Part model, mm, in its own coordinate system. Face numbers are marked on the shaded views. A direction names the side the tool comes from. Give positions to 0.01 mm unless a question says otherwise; leave off trailing zeros. Order: outer loops, then holes, each group sorted by start corner. A loop starts at its lowest first (then second) coordinate and runs counter-clockwise, first axis right, second up. Notation, with made-up numbers: (38, 68) - (47, 68) arc R23 cw to (47, 85) - close; hole circle Ø9 at (43, -29). An arc over 180 degrees is marked (long way). Use one line per item in the form item = value. Start each with the question number.
1. Band-saw the part on C-C, the plane y = -213. List the corners of the cut face in (x, z), plus the area to 3 significant figures.
2. Pin check, flat tips, straight feed: P1, Ø5.5, axis at x = 197.55, z = 3.2, coming from the -Y side; P2, Ø14.5, axis at x = 167.5, y = -180.5, coming from the +Z side; P3, Ø3, axis at y = -223.5, z = 9, coming from the -X side; P4, Ø8.5, axis at x = 88.5, z = 4.5, coming from the -Y side. Stop position of each tip, or through.
3. Band-saw the part on A-A, the plane x = 31. List the corners of the cut face in (y, z), plus the area to 3 significant figures.
4. Band-saw the part on B-B, the plane z = 8.5. State how many separate pieces and enclosed holes the cut face has, plus the area to 3 significant figures.
5. Pull direction X, two halves, no side cores. Call the marked faces 1, 2, 3 and 4: +X half, -X half, draft (parallel to the pull), parting line (faces both ways), or undercut.
6. Drill centre lines: line 1 (Z direction, x = 31, y = -188); line 2 (Z direction, x = 148.35, y = -226.6); line 3 (Y direction, x = 75, z = 7.5). Where is each one in solid material? Low to high.
7. Band-saw the part on D-D, the plane z = 20.25. List the corners of the cut face in (x, y), plus the area to 4 significant figures.
8. Tool access for the marked faces 5 and 6: list every direction of +Z, -Z, +X, -X, +Y, -Y with a clear straight run to the whole face (end or side of a thin tool).
from build123d import *

# Parameters (mm, degrees)
PAD067_DEPTH           = 10
PAD068_DEPTH           = 6
PAD072_DEPTH           = 14
CYLINDER038_R          = 2.2
CYLINDER038_DEPTH      = 26
CYLINDER038_ROLL_ANGLE = -90
ARRAY012_X_COUNT       = 2
ARRAY012_X_PITCH       = 8
ARRAY012_Z_COUNT       = 2
ARRAY012_Z_PITCH       = 9
BOX047_W               = 24
BOX047_H               = 10
BOX047_DEPTH           = 17
SKETCH056_R            = 3
PAD057_DEPTH           = 9
BOX048_W               = 35
BOX048_H               = 15
BOX048_DEPTH           = 20
BOX044_W               = 23
BOX044_H               = 3
BOX044_DEPTH           = 20
SKETCH049_R            = 3
PAD050_DEPTH           = 4
SKETCH050_R            = 3
PAD051_DEPTH           = 4
BOX043_W               = 20
BOX043_H               = 17
BOX043_DEPTH           = 10
FILLET017_R            = 1
FILLET017_ROLL_ANGLE   = 90
FILLET018_1_R          = 2
FILLET018_2_R          = 1
BOX042_W               = 167
BOX042_H               = 10
BOX042_DEPTH           = 17
CYLINDER037_R          = 2.2
CYLINDER037_DEPTH      = 18
CYLINDER037_ROLL_ANGLE = -90
ARRAY011_X_COUNT       = 2
ARRAY011_X_PITCH       = 49.2
ARRAY011_Z_COUNT       = 2
ARRAY011_Z_PITCH       = 10.3
PAD053_DEPTH           = 6
PAD052_DEPTH           = 10
CHAMFER007_SIZE        = 3
FILLET023_R            = 1
CHAMFER009_SIZE        = 7.5
PAD066_DEPTH           = 10


with BuildPart() as obj1:
    # Sketch067 → Pad067 (new body)
    with BuildSketch(Plane(origin=(142.7, 11, 18.5), x_dir=(0, 0, -1), z_dir=(1, 0, 0))):
        Polygon((0, 0), (0, 3), (3, 0), align=None)
    extrude(amount=PAD067_DEPTH)


with BuildPart() as obj2:
    # Sketch068 → Pad068 (new body)
    with BuildSketch(Plane(origin=(152.7, 45.8, 18.5), x_dir=(0, -1, 0), z_dir=(0, 0, 1))):
        Polygon((0, 0), (0, 3), (3, 0), align=None)
    extrude(amount=PAD068_DEPTH)


with BuildPart() as obj3:
    # Sketch065 → Pad072 (new body)
    with BuildSketch(Plane(origin=(152.7, 11, 17), x_dir=(1, 0, 0), z_dir=(0, -1, 0))):
        Polygon((0, 0), (0, 7), (7, 0), align=None)
    extrude(amount=PAD072_DEPTH)


with BuildPart() as obj4:
    # Cylinder038 → Cylinder038 (new body)
    with BuildSketch(Plane.XY):
        Circle(CYLINDER038_R)
    extrude(amount=CYLINDER038_DEPTH)


with BuildPart() as obj4_1:
    # Cylinder038 roll: moved
    add(obj4.part.rotate(Axis((0, 0, 0), (1, 0, 0)), CYLINDER038_ROLL_ANGLE))


with BuildPart() as obj4_2:
    # Cylinder038 placement: moved
    add(obj4_1.part.moved(Location((202, 0, 4))))

    # Array012 X: obj4_2


with BuildPart() as obj4_3:
    add(obj4_2.part)
    with Locations(*[(i * ARRAY012_X_PITCH, 0, 0) for i in range(1, ARRAY012_X_COUNT)]):
        add(obj4_2.part)

    # Array012 Z: obj4_2


with BuildPart() as obj4_4:
    add(obj4_3.part)
    with Locations(*[(0, 0, i * ARRAY012_Z_PITCH) for i in range(1, ARRAY012_Z_COUNT)]):
        add(obj4_3.part)


with BuildPart() as obj4_5:
    # Array012 placement: moved
    add(obj4_4.part.moved(Location((-171, -5, 0))))


with BuildPart() as obj5:
    # Box047 → Box047 (new body)
    with BuildSketch(Plane(origin=(26, 6, 0), x_dir=(1, 0, 0), z_dir=(0, 0, 1))):
        with Locations((12, 5)):
            Rectangle(BOX047_W, BOX047_H)
    extrude(amount=BOX047_DEPTH)


with BuildPart() as obj6:
    # Sketch056 → Pad057 (new body)
    with BuildSketch(Plane(origin=(50, 6, 0), x_dir=(1, 0, 0), z_dir=(0, -1, 0))):
        with BuildLine():
            Line((0, 17), (-36, 17))
            ThreePointArc((-36, 17), (-44.500015, 8.5), (-36, 0))
            Line((-36, 0), (0, 0))
            Line((0, 0), (0, 17))
        make_face()
        with Locations((-36.000015, 8.5)):
            Circle(SKETCH056_R, mode=Mode.SUBTRACT)
    extrude(amount=PAD057_DEPTH)


with BuildPart() as obj7:
    # Box048 → Box048 (new body)
    with BuildSketch(Plane(origin=(-2, -5, 0), x_dir=(1, 0, 0), z_dir=(0, 0, 1))):
        with Locations((17.5, 7.5)):
            Rectangle(BOX048_W, BOX048_H)
    extrude(amount=BOX048_DEPTH)


with BuildPart() as obj8:
    # Box044 → Box044 (new body)
    with BuildSketch(Plane(origin=(80.5, 1, 0), x_dir=(1, 0, 0), z_dir=(0, 0, 1))):
        with Locations((11.5, 1.5)):
            Rectangle(BOX044_W, BOX044_H)
    extrude(amount=BOX044_DEPTH)


with BuildPart() as obj9:
    # Sketch049 → Pad050 (new body)
    with BuildSketch(Plane.XY):
        with BuildLine():
            Line((0, 17), (20, 17))
            ThreePointArc((20, 0), (28.500019, 8.5), (20, 17))
            Line((20, 0), (0, 0))
            Line((0, 0), (0, 17))
        make_face()
        with Locations((20.000019, 8.5)):
            Circle(SKETCH049_R, mode=Mode.SUBTRACT)
    extrude(amount=PAD050_DEPTH)


with BuildPart() as obj10:
    # Sketch050 → Pad051 (new body)
    with BuildSketch(Plane.XY.offset(14)):
        with BuildLine():
            Line((0, 17), (20, 17))
            ThreePointArc((20, 0), (28.500019, 8.5), (20, 17))
            Line((20, 0), (0, 0))
            Line((0, 0), (0, 17))
        make_face()
        with Locations((20.000019, 8.5)):
            Circle(SKETCH050_R, mode=Mode.SUBTRACT)
    extrude(amount=PAD051_DEPTH)


with BuildPart() as obj11:
    # Box043 → Box043 (new body)
    with BuildSketch(Plane(origin=(-16, 0, 4), x_dir=(1, 0, 0), z_dir=(0, 0, 1))):
        with Locations((10, 8.5)):
            Rectangle(BOX043_W, BOX043_H)
    extrude(amount=BOX043_DEPTH)

    # Fusion009003048: union obj9, obj10
    add(obj9.part)
    add(obj10.part)

    # Fillet017
    fillet017_edges = [obj11.edges().sort_by_distance(p)[0] for p in [
        (0, 8.5, 18),
        (-16, 0, 9),
        (-16, 17, 9),
        (0, 8.5, 0),
    ]]
    fillet(fillet017_edges, radius=FILLET017_R)


with BuildPart() as obj11_1:
    # Fillet017 roll: moved
    add(obj11.part.rotate(Axis((0, 0, 0), (1, 0, 0)), FILLET017_ROLL_ANGLE))


with BuildPart() as obj11_2:
    # Fillet017 placement: moved
    add(obj11_1.part.moved(Location((16, 15, 0))))

    # Fillet018 1
    fillet018_1_edges = [obj11_2.edges().sort_by_distance(p)[0] for p in [
        (16, 1, 8.5),
        (16, 11, 8.5),
    ]]
    fillet(fillet018_1_edges, radius=FILLET018_1_R)

    # Fillet018 2
    fillet018_2_edges = [obj11_2.edges().sort_by_distance(p)[0] for p in [
        (20, 1, 8.5),
        (20, 11, 8.5),
    ]]
    fillet(fillet018_2_edges, radius=FILLET018_2_R)


with BuildPart() as obj11_3:
    # Fillet018 placement: moved
    add(obj11_2.part.moved(Location((149, 0, 0))))


with BuildPart() as obj12:
    # Box042 → Box042 (new body)
    with BuildSketch(Plane(origin=(0, -3, 0), x_dir=(1, 0, 0), z_dir=(0, 0, 1))):
        with Locations((83.5, 5)):
            Rectangle(BOX042_W, BOX042_H)
    extrude(amount=BOX042_DEPTH)

    # Fusion009003049: union obj11
    add(obj11_3.part)

    # Cut038: cut obj8
    add(obj8.part, mode=Mode.SUBTRACT)


with BuildPart() as obj13:
    # Cylinder037 → Cylinder037 (new body)
    with BuildSketch(Plane.XY):
        Circle(CYLINDER037_R)
    extrude(amount=CYLINDER037_DEPTH)


with BuildPart() as obj13_1:
    # Cylinder037 roll: moved
    add(obj13.part.rotate(Axis((0, 0, 0), (1, 0, 0)), CYLINDER037_ROLL_ANGLE))


with BuildPart() as obj13_2:
    # Cylinder037 placement: moved
    add(obj13_1.part.moved(Location((150.075, 41, 13.5))))

    # Array011 X: obj13_2


with BuildPart() as obj13_3:
    add(obj13_2.part)
    with Locations(*[(i * ARRAY011_X_PITCH, 0, 0) for i in range(1, ARRAY011_X_COUNT)]):
        add(obj13_2.part)

    # Array011 Z: obj13_2


with BuildPart() as obj13_4:
    add(obj13_3.part)
    with Locations(*[(0, 0, -i * ARRAY011_Z_PITCH) for i in range(1, ARRAY011_Z_COUNT)]):
        add(obj13_3.part)


with BuildPart() as obj14:
    # Sketch052 → Pad053 (new body)
    with BuildSketch(Plane(origin=(10, 54.8, 0), x_dir=(1, 0, 0), z_dir=(0, -1, 0))):
        Polygon((0, 18.5), (0, 24.5), (50.5, 24.5), (50.5, 0), (40.5, 0), (40.5, 18.5), align=None)
    extrude(amount=PAD053_DEPTH)


with BuildPart() as obj15:
    # Sketch051 → Pad052 (new body)
    with BuildSketch(Plane.YZ):
        Polygon((14, 0), (0, 0), (0, 24.5), (54.8, 24.5), (54.8, 0), (48.8, 0), (48.8, 18.5), (14, 18.5), align=None)
    extrude(amount=PAD052_DEPTH)

    # Fusion009003050: union obj14
    add(obj14.part)


with BuildPart() as obj15_1:
    # Fusion009003050 placement: moved
    add(obj15.part.moved(Location((144.425, -3, 0))))

    # Cut037: cut obj13
    add(obj13_4.part, mode=Mode.SUBTRACT)


with BuildPart() as obj15_2:
    # Cut037 placement: moved
    add(obj15_1.part.moved(Location((-1.725, 0, 0))))

    # Fusion009003051: union obj12
    add(obj12.part)

    # Chamfer007
    chamfer007_edges = [obj15_2.edges().sort_by_distance(p)[0] for p in [
        (142.7, 7, 8.5),
    ]]
    chamfer(chamfer007_edges, length=CHAMFER007_SIZE)

    # Cut039: cut obj7
    add(obj7.part, mode=Mode.SUBTRACT)

    # Fusion009003053: union obj6
    add(obj6.part)

    # Fusion009003054: union obj5
    add(obj5.part)

    # Cut040: cut obj4
    add(obj4_5.part, mode=Mode.SUBTRACT)

    # Fillet023
    fillet023_edges = [obj15_2.edges().sort_by_distance(p)[0] for p in [
        (50, 16, 8.5),
        (26, 11, 0),
        (26, 11, 17),
    ]]
    fillet(fillet023_edges, radius=FILLET023_R)

    # Chamfer009
    chamfer009_edges = [obj15_2.edges().sort_by_distance(p)[0] for p in [
        (50, 7, 8.5),
    ]]
    chamfer(chamfer009_edges, length=CHAMFER009_SIZE)


with BuildPart() as femur_izquierdo_full001:
    # Sketch066 → Pad066 (new body)
    with BuildSketch(Plane(origin=(142.7, -3, 17), x_dir=(-1, 0, 0), z_dir=(0, 1, 0))):
        Polygon((0, 0), (0, 7), (7, 0), align=None)
    extrude(amount=PAD066_DEPTH)

    # Fusion009003066: union obj1, obj2, obj3, obj15
    add(obj1.part)
    add(obj2.part)
    add(obj3.part)
    add(obj15_2.part)


with BuildPart() as femur_derecha_full:
    # Part__Mirroring012: instance of Femur_izquierdo_full001
    add(femur_izquierdo_full001.part.mirror(Plane(origin=(0, 0, 0), x_dir=(1, 0, 0), z_dir=(0, 1, 0))))


with BuildPart() as femur_derecha_full_1:
    # Part__Mirroring012 placement: moved
    add(femur_derecha_full.part.moved(Location((0, -178, 0))))


solid = femur_derecha_full_1.part
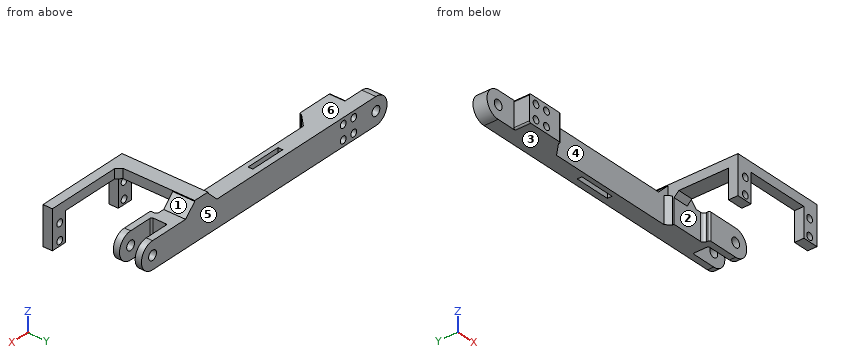
From the geometry:
q1.outline = (142.7, 18.5) - (152.7, 18.5) - (152.7, 24.5) - (142.7, 24.5) - close
q1.area = 60.0 mm²
q2.P1 = -229.8
q2.P2 = 17
q2.P3 = 142.7
q2.P4 = -185
q3.outline = (-194, 0) - (-175, 0) - (-175, 1.8) - (-194, 1.8) - close; (-194, 6.2) - (-175, 6.2) - (-175, 10.8) - (-194, 10.8) - close; (-194, 15.2) - (-175, 15.2) - (-175, 17) - (-194, 17) - close
q3.area = 156 mm²
q4.separate_pieces = 6
q4.enclosed_holes = 1
q4.area = 2,130 mm²
q5.face_1 = +X half
q5.face_2 = undercut
q5.face_3 = draft
q5.face_4 = undercut
q6.line_1 = 0 to 1.8, 6.2 to 10.8, 15.2 to 17
q6.line_2 = 0 to 1, 5.4 to 11.3, 15.7 to 24.5
q6.line_3 = -185 to -175
q7.outline = (138.95, -185) - (142.7, -185) - (142.7, -229.8) - (203.2, -229.8) - (203.2, -223.8) - (155.7, -223.8) - (152.7, -220.8) - (152.7, -189) - (156.45, -189) - (156.45, -175) - (138.95, -175) - close
q7.area = 945.5 mm²
q8.face_5 = +Z, -Z, +X, -X, +Y
q8.face_6 = +Z, -X, +Y, -Y
